from build123d import *

# Parameters (mm, degrees)
SKETCH2_R                = 101.6
SKETCH2_R_2              = 63.5
BOSS_EXTRUDE1_DEPTH      = 114.3
BOSS_EXTRUDE1_DEPTH_BACK = 2.54
FILLET1_R                = 12.7
SKETCH4_R                = 63.5
BOSS_EXTRUDE2_DEPTH      = 6.35
BOSS_EXTRUDE2_DEPTH_BACK = 6.35
SKETCH13_R               = 6.35
CUT_EXTRUDE1_DEPTH       = 50.53
CUT_EXTRUDE1_DEPTH_BACK  = 68.3100001


with BuildPart() as part:
    # Sketch2 → Boss-Extrude1 (new body, two sides)
    with BuildSketch(Plane.XY) as boss_extrude1_sk:
        Circle(SKETCH2_R)
        Circle(SKETCH2_R_2, mode=Mode.SUBTRACT)
    extrude(amount=BOSS_EXTRUDE1_DEPTH)
    extrude(boss_extrude1_sk.sketch, amount=-BOSS_EXTRUDE1_DEPTH_BACK)

    # Fillet1
    fillet1_edges = [part.edges().sort_by_distance(p)[0] for p in [
        (-101.6, 0, -2.54),
        (-63.5, 0, -2.54),
        (-101.6, 0, 114.3),
        (-63.5, 0, 114.3),
    ]]
    fillet(fillet1_edges, radius=FILLET1_R)

    # Sketch4 → Boss-Extrude2 (add, two sides)
    with BuildSketch(Plane(origin=(0, 0, 55.88), x_dir=(-1, 0, 0), z_dir=(0, 0, -1))) as boss_extrude2_sk:
        Circle(SKETCH4_R)
    extrude(amount=BOSS_EXTRUDE2_DEPTH)
    extrude(boss_extrude2_sk.sketch, amount=-BOSS_EXTRUDE2_DEPTH_BACK)

    # Sketch13 → Cut-Extrude1 (cut, two sides)
    with BuildSketch(Plane.XY.offset(64.77)) as cut_extrude1_sk:
        Circle(SKETCH13_R)
        with Locations((-35.941, 0)):
            Circle(SKETCH13_R)
        with Locations((-11.106379795, 34.181922252)):
            Circle(SKETCH13_R)
        with Locations((29.076879795, 21.125589753)):
            Circle(SKETCH13_R)
        with Locations((29.076879795, -21.125589753)):
            Circle(SKETCH13_R)
        with Locations((-11.106379795, -34.181922252)):
            Circle(SKETCH13_R)
    extrude(amount=CUT_EXTRUDE1_DEPTH, mode=Mode.SUBTRACT)
    extrude(cut_extrude1_sk.sketch, amount=-CUT_EXTRUDE1_DEPTH_BACK, mode=Mode.SUBTRACT)


solid = part.part
Source: CAD feature listing. Evaluate the final solid. Frame: model axes, mm. A direction names the side the tool comes from. Give positions to 0.01 mm unless a question says otherwise; leave off trailing zeros. Write each loop counter-clockwise with the first axis right and the second up, starting at its lowest first coordinate (ties: lowest second). Pieces come first, ordered by that corner, then holes. Notation, with made-up numbers: (42.25, -26.75) - (82.25, -26.75) arc R10 ccw to (82.25, -19.75) - close; hole circle Ø7 at (-14.5, 70.25). An arc over 180 degrees is marked (long way). Write item = value, one per line. Start each with the question number.
Q1. Reachability of faces 1 (the cylindrical face through (-11.933, -27.886, 55.969)), 2 (the flat face through (1, -13, 62.23)), 3 (the flat face through (1, -13, 49.53)) from +Z, -Z, +X, -X, +Y, -Y: full face, straight path, thin tool, end or side. Return the list, or none.
Q2. Draft query along X for faces 4 (the flat face through (65.4, 39.9, -2.54)), 5 (the cylindrical face through (-17.45, 34.46, 55.97)), 6 (the cylindrical face through (-22.025, -99.184, 56.52)). Return one class per face: +X half, -X half, draft (parallel to the pull), parting line (faces both ways), or undercut.
Q3. Cut plane B-B, the plane z = 15. Return loops of the section in (x, y), then the cut area to 3 significant figures.
Q4. Cut plane A-A, the plane y = 0. Give the number of separate pieces and of enclosed holes in the cut face, then the cut area to 3 significant figures.
Q5. Pin query (flat end, axial travel): pin 1 Ø5 at (x, z) = (33, 28) entering from +Y; pin 2 Ø8 at (x, y) = (-3.5, -12) entering from +Z; pin 3 Ø3 at (x, z) = (-36.5, 71.5) entering from +Y. Return the tip coordinate at first contact, or that it passes through.
Q6. Material intervals for probe 1 along Y at (x, z) = (-0.5, 102); probe 2 along Y at (x, z) = (0, 58); probe 3 along Z at (x, y) = (39.5, -2), sorted ascending.
Q7. Cut plane D-D, the plane z = 54. Return loops of the section in (x, y), then the cut area to 3 significant figures.
Computed values:
q1.face_1 = +Z, -Z
q1.face_2 = +Z
q1.face_3 = -Z
q2.face_4 = draft
q2.face_5 = undercut
q2.face_6 = parting line
q3.outline = circle Ø203.2 at (0, 0); hole circle Ø127 at (0, 0)
q3.area = 19,800 mm²
q4.separate_pieces = 3
q4.enclosed_holes = 0
q4.area = 9,920 mm²
q5.pin_1 = 96.91
q5.pin_2 = 62.23
q5.pin_3 = 95.38
q6.probe_1 = -101.59 to -63.5, 63.5 to 101.59
q6.probe_2 = -101.6 to -6.35, 6.35 to 101.6
q6.probe_3 = 49.53 to 62.23
q7.outline = circle Ø203.2 at (0, 0); hole circle Ø12.7 at (-35.94, 0); hole circle Ø12.7 at (-11.11, -34.18); hole circle Ø12.7 at (-11.11, 34.18); hole circle Ø12.7 at (0, 0); hole circle Ø12.7 at (29.08, -21.13); hole circle Ø12.7 at (29.08, 21.13)
q7.area = 31,700 mm²
